Geometry check sheet. Reference: the model listing, model coordinates, mm. A direction names the side the tool comes from. Coordinates: 2 decimals unless noted, no trailing zeros. Write each loop counter-clockwise with the first axis right and the second up, starting at its lowest first coordinate (ties: lowest second). Pieces come first, ordered by that corner, then holes. Notation, with made-up numbers: M -12.5,-13 L 12.5,-13 A33 ccw 12.5,21 Z; hole C 7.5,79.5 d5. An arc over 180 degrees is marked long. Write each question's results on one line, items separated by ' | '.
```python
from build123d import *

# Parameters (mm, degrees)
F1_DEPTH = 177.8
F4_DEPTH = 177.801
F5_W     = 25.4
F5_H     = 76.2
F5_H_2   = 63.5
F6_DEPTH = 25.4
F7_R     = 3.175
F8_DEPTH = 25.4
F7_R_2   = 6.223
F9_DEPTH = 6.35


# Not quite as in the source:
# - a feature names something its author has since deleted; it is built from what else it names


with BuildPart() as f1:
    # F0 (on Front) → F1 (new body)
    with BuildSketch(Plane.XZ):
        with BuildLine():
            ThreePointArc((-38.1, 80.3218525683), (-47.519048812, -75.1342132454), (88.9, 0))
            ThreePointArc((88.9, 0), (75.1342132454, 47.519048812), (38.1, 80.3218525683))
            ThreePointArc((38.1, 80.3218525683), (19.5268700344, 86.7289533354), (0, 88.9))
            ThreePointArc((0, 88.9), (-19.5268700344, 86.7289533354), (-38.1, 80.3218525683))
        make_face()
        with BuildLine():
            ThreePointArc((0, 88.9), (19.5268700344, 86.7289533354), (38.1, 80.3218525683))
            Line((38.1, 80.3218525683), (38.1, 88.9))
            Line((38.1, 88.9), (0, 88.9))
        make_face()
        with BuildLine():
            Line((-38.1, 88.9), (-38.1, 80.3218525683))
            ThreePointArc((-38.1, 80.3218525683), (-19.5268700344, 86.7289533354), (0, 88.9))
            Line((0, 88.9), (-38.1, 88.9))
        make_face()
    extrude(amount=-F1_DEPTH)

    # F3 (on face) → F4 (cut, through all)
    with BuildSketch(Plane.XZ):
        with BuildLine():
            Line((-76.2, 0), (0, 0))
            Line((0, 0), (0, 76.2))
            ThreePointArc((0, 76.2), (-4.4029328075, 77.974338005), (-6.3453015162, 82.3057692308))
            ThreePointArc((-6.3453015162, 82.3057692308), (-58.3716647869, 58.3716647869), (-82.3057692308, 6.3453015162))
            ThreePointArc((-82.3057692308, 6.3453015162), (-77.974338005, 4.4029328075), (-76.2, 0))
        make_face()
        with BuildLine():
            Line((0, -76.2), (0, 0))
            Line((0, 0), (-76.2, 0))
            ThreePointArc((-76.2, 0), (-77.974338005, -4.4029328075), (-82.3057692308, -6.3453015162))
            ThreePointArc((-82.3057692308, -6.3453015162), (-58.3716647869, -58.3716647869), (-6.3453015162, -82.3057692308))
            ThreePointArc((-6.3453015162, -82.3057692308), (-4.4029328075, -77.974338005), (0, -76.2))
        make_face()
        with BuildLine():
            Line((0, 76.2), (0, 0))
            Line((0, 0), (76.2, 0))
            ThreePointArc((76.2, 0), (77.974338005, 4.4029328075), (82.3057692308, 6.3453015162))
            ThreePointArc((82.3057692308, 6.3453015162), (58.3716647869, 58.3716647869), (6.3453015162, 82.3057692308))
            ThreePointArc((6.3453015162, 82.3057692308), (4.4029328075, 77.974338005), (0, 76.2))
        make_face()
        with BuildLine():
            Line((76.2, 0), (0, 0))
            Line((0, 0), (0, -76.2))
            ThreePointArc((0, -76.2), (4.4029328075, -77.974338005), (6.3453015162, -82.3057692308))
            ThreePointArc((6.3453015162, -82.3057692308), (58.3716647869, -58.3716647869), (82.3057692308, -6.3453015162))
            ThreePointArc((82.3057692308, -6.3453015162), (77.974338005, -4.4029328075), (76.2, 0))
        make_face()
    extrude(amount=-F4_DEPTH, mode=Mode.SUBTRACT)

    # F5 (on face) → F6 (cut)
    with BuildSketch(Plane.XY.offset(88.9)):
        with Locations((-19.05, 50.8)):
            Rectangle(F5_W, F5_H)
        with Locations((19.05, 50.8)):
            Rectangle(F5_W, F5_H)
        with Locations((19.05, 133.35)):
            Rectangle(F5_W, F5_H_2)
        with Locations((-19.05, 133.35)):
            Rectangle(F5_W, F5_H_2)
    extrude(amount=-F6_DEPTH, mode=Mode.SUBTRACT)

    # F7 (on face) → F8 (cut)
    with BuildSketch(Plane.XY.offset(88.9)):
        with Locations((-31.75, 95.25)):
            Circle(F7_R)
        with Locations((-31.75, 171.45)):
            Circle(F7_R)
        with Locations((31.75, 171.45)):
            Circle(F7_R)
        with Locations((31.75, 95.25)):
            Circle(F7_R)
        with Locations((31.75, 6.35)):
            Circle(F7_R)
        with Locations((-31.75, 6.35)):
            Circle(F7_R)
    extrude(amount=-F8_DEPTH, mode=Mode.SUBTRACT)

    # F7 (on face) → F9 (join)
    with BuildSketch(Plane.XY.offset(88.9)):
        with Locations((0, 171.45)):
            Circle(F7_R_2)
        with Locations((0, 6.35)):
            Circle(F7_R_2)
    extrude(amount=F9_DEPTH)


solid = f1.part
```
Q1. Scan lines: probe 1 along X at (y, z) = (171.45, 83.75) (3 decimals); probe 2 along X at (y, z) = (171, 77); probe 3 along Y at (x, z) = (-31, 79). Record each from-to range of solid material in increasing order.
Geometry check:
probe 1: x = -38.1 to -34.925, -28.575 to 28.575, 34.925 to 38.1 | probe 2: x = -44.43 to -34.89, -3.09 to 3.09, 34.89 to 44.43 | probe 3: y = 0 to 3.26, 9.44 to 12.7, 88.9 to 92.16, 98.34 to 101.6, 165.1 to 168.36, 174.54 to 177.8
Q2. Depth check by flat-ended pin: P1, Ø7.5, axis at x = 31.75, y = 6.35, coming from the +Z side; P2, Ø5, axis at x = 31.75, y = 95.25, coming from the +Z side; P3, Ø8, axis at y = 74, z = 59.5, coming from the -X side. Enter the tip coordinate at first touch or a pass-through.
Geometry check:
P1: stops at z = 88.9 | P2: stops at z = -75.11 | P3: stops at x = -69.45
Q3. Access from +Z, -Z, +X, -X, +Y, -Y to the whole of each face (thin tool, end or side, straight path). Record for faces 1 (the flat face through (0, 172, 95.25)), 2 (the flat face through (31.75, 133, 83)).
Geometry check:
face 1: +Z, +X, -X, +Y, -Y | face 2: +Z
Q4. Sectioned sample at B-B on x = 25. Record the cut outline in (y, z).
Geometry check:
outline: M 0,-85.31 L 177.8,-85.31 L 177.8,-78.67 L 0,-78.67 Z; M 0,78.67 L 12.7,78.67 L 12.7,88.9 L 0,88.9 Z; M 88.9,78.67 L 101.6,78.67 L 101.6,88.9 L 88.9,88.9 Z; M 165.1,78.67 L 177.8,78.67 L 177.8,88.9 L 165.1,88.9 Z
Q5. Sectioned sample at C-C on z = -30. Record the cut outline in (x, y).
Geometry check:
outline: M -83.69,0 L -76.91,0 L -76.91,177.8 L -83.69,177.8 Z; M 76.91,0 L 83.69,0 L 83.69,177.8 L 76.91,177.8 Z
Q6. Sectioned sample at D-D on x = -51.5. Record the cut outline in (y, z), and give its area (3 significant figures).
Geometry check:
outline: M 0,-72.46 L 177.8,-72.46 L 177.8,-64.52 L 0,-64.52 Z; M 0,64.52 L 177.8,64.52 L 177.8,72.46 L 0,72.46 Z | area: 2,830 mm2
